Could you check a few things on this model? Use its own coordinates, in mm. A direction names the side the tool comes from. Round coordinates to 2 decimals unless told otherwise and drop trailing zeros. Loops run counter-clockwise (first coordinate to the right, second up) from the corner with the lowest first, then second, coordinate; pieces in that order, holes last. Notation, with made-up numbers: (-18, 68) -> (-12, 68) arc R23 cw to (-12, 86) -> close; hole circle Ø6 at (1, 12.5). An arc over 180 degrees is marked (long way). One line per item, written item: value.
from build123d import *

# Parameters (mm, degrees)
SKETCH1_W                      = 15.875
SKETCH1_H                      = 46.0375
BOSS_EXTRUDE1_DEPTH            = 0.5953125
SKETCH2_R                      = 2.778125
SKETCH2_R_2                    = 1.5875
BOSS_EXTRUDE2_DEPTH            = 23.01875
CUT_EXTRUDE1_DEPTH             = 26.870801526
CUT_EXTRUDE1_DEPTH_BACK        = 26.870801526
SKETCH3_W                      = 6.35
SKETCH3_H                      = 22.225
F_3_16_0_1875_DIAMETER_HOLE1_D = 4.7625


with BuildPart() as part:
    # Sketch1 → Boss-Extrude1 (new, symmetric)
    with BuildSketch(Plane.XY):
        Rectangle(SKETCH1_W, SKETCH1_H)
    extrude(amount=BOSS_EXTRUDE1_DEPTH, both=True)

    # Sketch2 → Boss-Extrude2 (add, symmetric)
    with BuildSketch(Plane(origin=(0, 0, 0), x_dir=(1, 0, 0), z_dir=(0, 1, 0))):
        with Locations((-7.9375, 2.1828125)):
            Circle(SKETCH2_R)
        with Locations(Location((-7.9375, 2.1828125, 0), (0, 0, 270))):
            Circle(SKETCH2_R_2, mode=Mode.SUBTRACT)
    extrude(amount=BOSS_EXTRUDE2_DEPTH, both=True)

    # Sketch3 → Cut-Extrude1 (cut, two sides: drawn at the far end of the back side and taken through both)
    with BuildSketch(Plane.XY.offset(-CUT_EXTRUDE1_DEPTH_BACK)):
        with Locations((-7.540625, 0)):
            Rectangle(SKETCH3_W, SKETCH3_H)
    extrude(amount=CUT_EXTRUDE1_DEPTH + CUT_EXTRUDE1_DEPTH_BACK, mode=Mode.SUBTRACT)

    # 3/16 (0.1875) Diameter Hole1 (through all)
    with Locations(Plane(origin=(0, 0, -0.5953125), x_dir=(-1, 0, 0), z_dir=(0, 0, -1))):
        with Locations((-1.5875, -19.05), (-1.5875, 0), (-1.5875, 19.05)):
            Hole(F_3_16_0_1875_DIAMETER_HOLE1_D / 2)


solid = part.part
(1) If we section it at C-C, the plane z = -4.3: Please give me the cut outline in (x, y), then the cut area to 3 significant figures.
Recorded:
outline: (-9.74, -23.02) -> (-6.14, -23.02) -> (-6.14, -11.11) -> (-9.74, -11.11) -> close; (-9.74, 11.11) -> (-6.14, 11.11) -> (-6.14, 23.02) -> (-9.74, 23.02) -> close
area: 85.7 mm²
(2) I'm going to push flat-ended pins straight in: pin 1 Ø11 at (x, y) = (-1, -2.5) entering from -Z; pin 2 Ø1 at (y, z) = (-0.5, 0) entering from -X. Where does each tip first touch, or does it pass through?
Recorded:
pin 1: z = -0.6
pin 2: x = -4.37
(3) For faces 1 (the face through (7.938, 0, 0)), 2 (the face through (-6, 11.112, -2)), which set-ups out of +Z, -Z, +X, -X, +Y, -Y let a thin tool reach every point of the face, with its end or its side?
Recorded:
face 1: +Z, -Z, +X, +Y, -Y
face 2: +Z, -Z, -X
(4) If I drill on L1, parallel to Y at x = -5.5, z = -1.4; L2, parallel to Z at x = -1, y = -2; L3, parallel to X at y = 9.5, z = -0.5, over which ranges is the centre line in solid material (lowest first)?
Recorded:
L1: -23.02 to -11.11, 11.11 to 23.02
L2: -0.6 to 0.6
L3: -4.37 to 7.94
(5) If we section it at A-A, the plane y = 19.05: Please give me the cut outline in (x, z) (1 decimal).
Recorded:
outline: (-7.9, 0.6) arc R2.8 ccw (long way) to (-5.7, -0.6) -> (-0.8, -0.6) -> (-0.8, 0.6) -> close; (4, -0.6) -> (7.9, -0.6) -> (7.9, 0.6) -> (4, 0.6) -> close; hole circle Ø3.2 at (-7.9, -2.2)
(6) Thinking about a two-plate mould opening in Z: for faces 3 (the face through (2.69, -21.16, 0.01)), 4 (the face through (-2, 0, 0.595)), 5 (the face through (-7.46, -17.15, -0.67)), which applies, released by +Z, released by -Z, zero draft, split by the parting line, or undercut?
Recorded:
face 3: zero draft
face 4: released by +Z
face 5: undercut
(7) If we section it at D-D, the plane x = 0.5: Please give me the cut outline in (y, z), then the cut area to 3 significant figures.
Recorded:
outline: (-23.02, -0.6) -> (-21.17, -0.6) -> (-21.17, 0.6) -> (-23.02, 0.6) -> close; (-16.93, -0.6) -> (-2.12, -0.6) -> (-2.12, 0.6) -> (-16.93, 0.6) -> close; (2.12, -0.6) -> (16.93, -0.6) -> (16.93, 0.6) -> (2.12, 0.6) -> close; (21.17, -0.6) -> (23.02, -0.6) -> (23.02, 0.6) -> (21.17, 0.6) -> close
area: 39.7 mm²
(8) If we section it at B-B, the plane y = 0: Please give me the cut outline in (x, z), then the cut area to 3 significant figures.
Recorded:
outline: (-4.37, -0.6) -> (-0.79, -0.6) -> (-0.79, 0.6) -> (-4.37, 0.6) -> close; (3.97, -0.6) -> (7.94, -0.6) -> (7.94, 0.6) -> (3.97, 0.6) -> close
area: 8.98 mm²
